```python
from build123d import *

# Parameters (mm, degrees)
SKETCH_W        = 50
SKETCH_H        = 21
PAD_DEPTH       = 10
SKETCH001_W     = 42.5
SKETCH001_H     = 10
POCKET_DEPTH    = 7
SKETCH002_R     = 1.6
POCKET001_DEPTH = 5
POCKET002_DEPTH = 7
SKETCH004_W     = 50
SKETCH004_H     = 7
POCKET003_DEPTH = 4.1
SKETCH005_R     = 1.6
POCKET004_DEPTH = 10.001


with BuildPart() as part:
    # Sketch → Pad (new body)
    with BuildSketch(Plane.XY):
        with Locations((25, 10.5)):
            Rectangle(SKETCH_W, SKETCH_H)
    extrude(amount=PAD_DEPTH)

    # Sketch001 (on Face6 of Pad) → Pocket (cut)
    with BuildSketch(Plane.XY.offset(10)):
        with Locations((25, 16)):
            Rectangle(SKETCH001_W, SKETCH001_H)
    extrude(amount=-POCKET_DEPTH, mode=Mode.SUBTRACT)

    # Sketch002 (on Face6 of Pocket) → Pocket001 (cut)
    with BuildSketch(Plane.XY.offset(3)):
        with Locations((9.5, 16.7)):
            Circle(SKETCH002_R)
        with Locations((40.5, 16.7)):
            Circle(SKETCH002_R)
    extrude(amount=-POCKET001_DEPTH, mode=Mode.SUBTRACT)

    # Sketch003 (on Face9 of Pocket001) → Pocket002 (cut)
    with BuildSketch(Plane.XZ):
        Polygon((4.9, 0), (20.1, 0), (17.6, 5.9), (7.4, 5.9), align=None)
        Polygon((29.9, 0), (45.1, 0), (42.6, 5.9), (32.4, 5.9), align=None)
    extrude(amount=-POCKET002_DEPTH, mode=Mode.SUBTRACT)

    # Sketch004 (on Face4 of Pocket002) → Pocket003 (cut)
    with BuildSketch(Plane.XY.offset(10)):
        with Locations((25, 3.5)):
            Rectangle(SKETCH004_W, SKETCH004_H)
    extrude(amount=-POCKET003_DEPTH, mode=Mode.SUBTRACT)

    # Sketch005 (on Face2 of Pocket003) → Pocket004 (cut, through all)
    with BuildSketch(Plane(origin=(0, 0, 0), x_dir=(1, 0, 0), z_dir=(0, 0, -1))):
        with Locations((25, -3.5)):
            Circle(SKETCH005_R)
    extrude(amount=-POCKET004_DEPTH, mode=Mode.SUBTRACT)


solid = part.part
```
Input: part model. Units: mm. Frame: model coordinates. A direction names the side the tool comes from. Round coordinates to 2 decimals unless told otherwise and drop trailing zeros. Write each loop counter-clockwise with the first axis right and the second up, starting at its lowest first coordinate (ties: lowest second). Pieces come first, ordered by that corner, then holes. Notation, with made-up numbers: M -38.5,-7.75 L 2.5,-7.75 A24 cw 2.5,3.25 Z; hole C -22,-18 d10. An arc over 180 degrees is marked long. Write each question's results on one line, items separated by ' | '.
Q1. Section query D-D (y = 3.5). Return loops of the section in (x, z), and give its area (3 significant figures).
Results:
outline: M 0,0 L 4.9,0 L 7.4,5.9 L 0,5.9 Z; M 17.6,5.9 L 20.1,0 L 23.4,0 L 23.4,5.9 Z; M 26.6,0 L 29.9,0 L 32.4,5.9 L 26.6,5.9 Z; M 42.6,5.9 L 45.1,0 L 50,0 L 50,5.9 Z | area: 126 mm^2
Q2. Access query for faces 1 (the face through (40.15, 15.14, 1.52)), 2 (the face through (3.75, 16, 7)), 3 (the face through (18.868, 3.451, 2.909)), 4 (the face through (4, 4, 5.9)), 5 (the face through (50, 13, 5)). Directions: +Z, -Z, +X, -X, +Y, -Y. A direction counts if a zero-diameter tool reaches every point of the face in a straight line with its end or side. Return the directions, or none.
Results:
face 1: +Z, -Z | face 2: +Z, +Y | face 3: -Z, -Y | face 4: +Z, +X, -X, -Y | face 5: +Z, -Z, +X, +Y, -Y
Q3. Draft query along Y for faces 6 (the face through (25, 13, 0)), 7 (the face through (7.9, 16.77, 1.52)), 8 (the face through (47, 0, 3)). Return one class per face: released by +Y, released by -Y, zero draft, split by the parting line, or undercut.
Results:
face 6: zero draft | face 7: undercut | face 8: released by -Y
Q4. Section query A-A (x = 40.5). Return loops of the section in (y, z).
Results:
outline: M 7,0 L 15.1,0 L 15.1,3 L 11,3 L 11,10 L 7,10 Z; M 18.3,0 L 21,0 L 21,3 L 18.3,3 Z
Q5. Section query B-B (y = 16.7). Return loops of the section in (x, z), and give its area (3 significant figures).
Results:
outline: M 0,0 L 7.9,0 L 7.9,3 L 3.75,3 L 3.75,10 L 0,10 Z; M 11.1,0 L 38.9,0 L 38.9,3 L 11.1,3 Z; M 42.1,0 L 50,0 L 50,10 L 46.25,10 L 46.25,3 L 42.1,3 Z | area: 183 mm^2
Q6. Line query: line 1 along Y through (x, z) = (40.5, 1.6); line 2 along X through (y, z) = (1, 3.75); line 3 along X through (y, z) = (5.25, 1). Output: solid intervals per line, ascending.
Results:
line 1: y = 7 to 15.1, 18.3 to 21 | line 2: x = 0 to 6.49, 18.51 to 31.49, 43.51 to 50 | line 3: x = 0 to 5.32, 19.68 to 30.32, 44.68 to 50
Q7. Pin query (flat end, axial travel): P1, Ø3.5, axis at x = 40.5, y = 16.7, coming from the -Z side; P2, Ø2, axis at x = 20, z = 6.5, coming from the +Y side; P3, Ø2, axis at x = 2, y = 3.5, coming from the +Z side; P4, Ø3.5, axis at x = 9.5, y = 16.7, coming from the +Z side. Return the tip coordinate at first contact, or that it passes through.
Results:
P1: stops at z = 0 | P2: stops at y = 11 | P3: stops at z = 5.9 | P4: stops at z = 3
Q8. Section query C-C (z = 6.5). Return loops of the section in (x, y).
Results:
outline: M 0,7 L 50,7 L 50,21 L 46.25,21 L 46.25,11 L 3.75,11 L 3.75,21 L 0,21 Z
